Drawing for the job (mm, zero at the part's lowest x, y, z). A direction names the side the tool comes from. Coordinates: 2 decimals unless noted, no trailing zeros. Write each loop counter-clockwise with the first axis right and the second up, starting at its lowest first coordinate (ties: lowest second). Pieces come first, ordered by that corner, then holes.
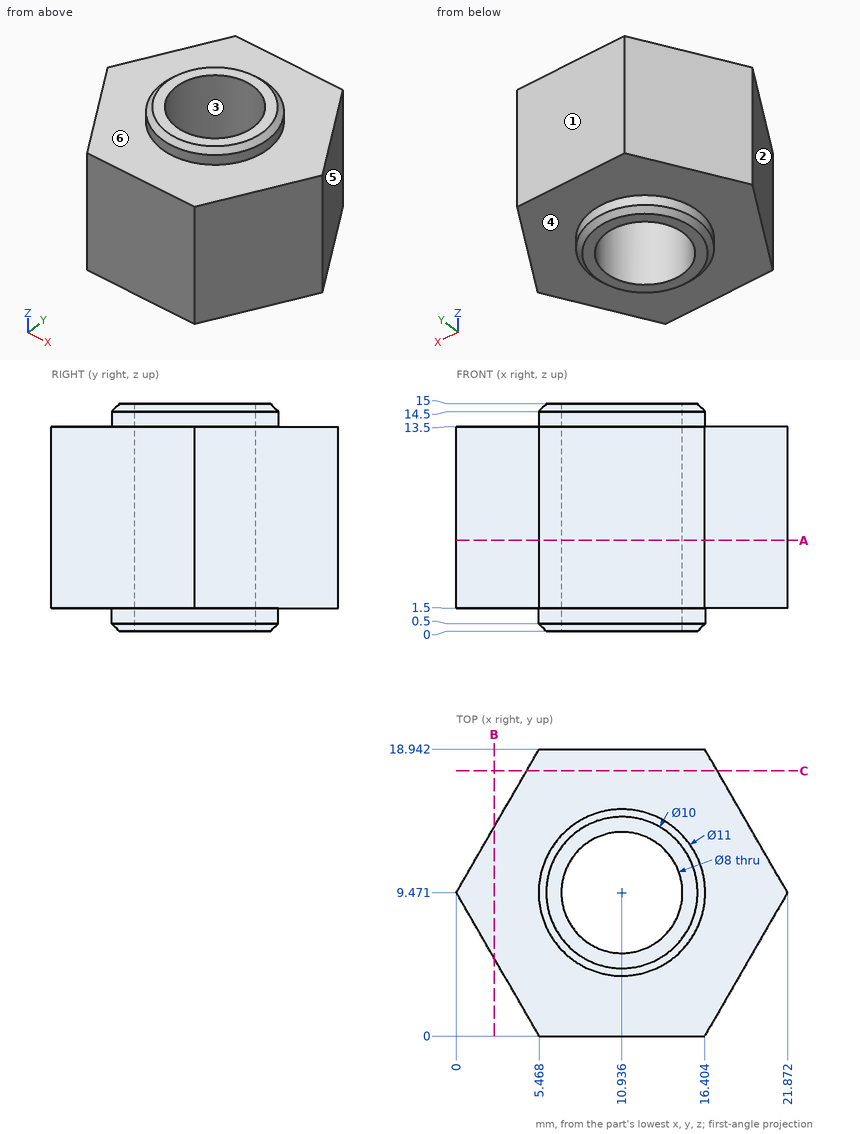
Item 1: Saw through at B-B, the plane x = 2.5. Write the cut outline in (y, z), and give its area (3 significant figures).
Item 2: Two-plate mould, pull along Y, no slides. Class the marked faces 1, 2, 3 and 4: +Y half, -Y half, draft (parallel to the pull), parting line (faces both ways), or undercut.
Item 3: Wall check: line 1 along Z through (x, y) = (12, 1.75); line 2 along X through (y, z) = (12, 13) (1 decimal); line 3 along X through (y, z) = (12.25, 13.75) (1 decimal). Give the ranges that are in metal, low to high.
Item 4: Saw through at C-C, the plane y = 17.5. Write the cut outline in (x, z) (1 decimal), and give its area (3 significant figures).
Item 5: Which spindle directions (+Z, -Z, +X, -X, +Y, -Y) get a long thin tool onto all of the face, cutting with end or side? Do the marked faces 5 and 6. Say none if no direction does.
Item 6: Saw through at A-A, the plane z = 6. Write the cut outline in (x, y) (1 decimal).
Item 7: Flat gauge pins, fed straight in: pin 1 Ø2 at (x, y) = (2.5, 10) entering from +Z; pin 2 Ø2 at (x, z) = (3, 8.5) entering from +Y; pin 3 Ø6.5 at (x, y) = (10.94, 9.47) entering from +Z; pin 4 Ø5 at (x, y) = (18, 4.5) entering from -Z. Where does each tip first touch, or does it go through?
Working result:
1. outline: (5.14, 1.5) - (13.8, 1.5) - (13.8, 13.5) - (5.14, 13.5) - close
1. area: 104 mm2
2. face 1: +Y half
2. face 2: -Y half
2. face 3: undercut
2. face 4: draft
3. line 1: z = 1.5 to 13.5
3. line 2: x = 1.5 to 7.8, 14 to 20.4
3. line 3: x = 6.2 to 8.1, 13.8 to 15.7
4. outline: (4.6, 1.5) - (17.2, 1.5) - (17.2, 13.5) - (4.6, 13.5) - close
4. area: 151 mm2
5. face 5: +Z, -Z, +X, +Y
5. face 6: +Z
6. outline: (0, 9.5) - (5.5, 0) - (16.4, 0) - (21.9, 9.5) - (16.4, 18.9) - (5.5, 18.9) - close; hole circle Ø8 at (10.9, 9.5)
7. pin 1: stops at z = 13.5
7. pin 2: stops at y = 16.4
7. pin 3: passes through
7. pin 4: stops at z = 1.5
